Geometry check sheet. Reference: the model listing, model coordinates, mm. Face numbers are marked on the shaded views. A direction names the side the tool comes from. Coordinates: 2 decimals unless noted, no trailing zeros. Loops run counter-clockwise (first coordinate to the right, second up) from the corner with the lowest first, then second, coordinate; pieces in that order, holes last.
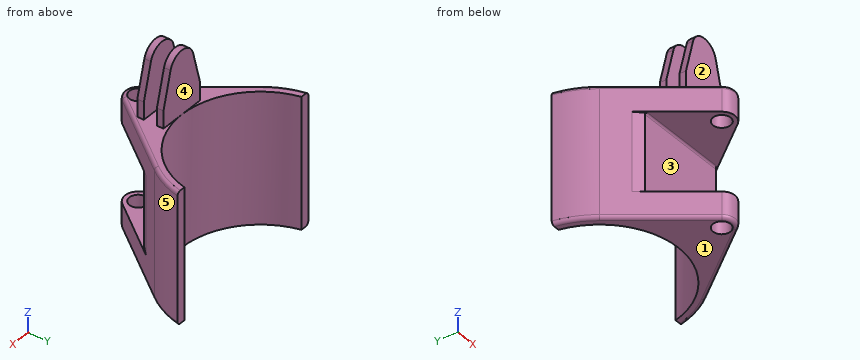
from build123d import *

# Parameters (mm, degrees)
SKETCH1_R             = 30
BOSS_EXTRUDE2_DEPTH   = 225
BOSS_EXTRUDE3_START   = 60
BOSS_EXTRUDE3_DEPTH   = 90
SKETCH3_W             = 257.405164054
SKETCH3_H             = 45
CUT_EXTRUDE1_DEPTH    = 151.9
SKETCH4_W             = 270
SKETCH4_H             = 367.4
CUT_EXTRUDE2_DEPTH    = 421.85
CHAMFER1_SIZE         = 6
CHAMFER1_SIZE2        = 32.008563289
CHAMFER1_EDGE_2_SIZE  = 6
CHAMFER1_EDGE_2_SIZE2 = 32.008563289
FILLET1_R             = 6
FILLET2_R             = 12


with BuildPart() as part:
    # Sketch1 → Boss-Extrude2 (new, symmetric)
    with BuildSketch(Plane.XY):
        with BuildLine():
            Line((238.377808514, 237.857142857), (35.756671277, -27.321428571))
            ThreePointArc((35.756671277, -27.321428571), (0, -45), (-35.756671277, -27.321428571))
            Line((-35.756671277, -27.321428571), (-238.377808514, 237.857142857))
            ThreePointArc((-238.377808514, 237.857142857), (-273.074997203, 295.782264138), (-293.938769134, 360))
            Line((-293.938769134, 360), (-263.248931622, 360))
            ThreePointArc((-263.248931622, 360), (0, 150), (263.248931622, 360))
            Line((263.248931622, 360), (293.938769134, 360))
            ThreePointArc((293.938769134, 360), (273.074997203, 295.782264138), (238.377808514, 237.857142857))
        make_face()
        Circle(SKETCH1_R, mode=Mode.SUBTRACT)
    extrude(amount=BOSS_EXTRUDE2_DEPTH, both=True)

    # Sketch2 → Boss-Extrude3 (add)
    with BuildSketch(Plane(origin=(0, 0, 0), x_dir=(1, 0, 0), z_dir=(0, 1, 0)).offset(BOSS_EXTRUDE3_START)):
        with BuildLine():
            Line((82.5, -225), (-82.5, -225))
            Line((-82.5, -225), (-82.5, -285))
            Line((-82.5, -285), (-50.709680046, -403.593320036))
            ThreePointArc((-50.709680046, -403.593320036), (0, -442.5), (50.709680046, -403.593320036))
            Line((50.709680046, -403.593320036), (82.5, -285))
            Line((82.5, -285), (82.5, -225))
        make_face()
    extrude(amount=BOSS_EXTRUDE3_DEPTH)

    # Sketch3 → Cut-Extrude1 (cut, symmetric)
    with BuildSketch(Plane(origin=(0, 0, 0), x_dir=(0, 0, -1), z_dir=(1, 0, 0))):
        with Locations((-353.702582027, 105)):
            Rectangle(SKETCH3_W, SKETCH3_H)
    extrude(amount=CUT_EXTRUDE1_DEPTH, both=True, mode=Mode.SUBTRACT)

    # Sketch4 → Cut-Extrude2 (cut, symmetric)
    with BuildSketch(Plane(origin=(0, 0, 0), x_dir=(0, 0, -1), z_dir=(1, 0, 0))):
        with Locations((0, -41.2)):
            Rectangle(SKETCH4_W, SKETCH4_H)
    extrude(amount=CUT_EXTRUDE2_DEPTH, both=True, mode=Mode.SUBTRACT)

    # Chamfer1
    chamfer1_edges = [part.edges().sort_by_distance(p)[0] for p in [
        (165.516066235, 142.5, 0),
    ]]
    chamfer1_side = [part.faces().sort_by_distance(p)[0] for p in [
        (0, 142.5, 0),
    ]]
    chamfer(chamfer1_edges, length=CHAMFER1_SIZE, length2=CHAMFER1_SIZE2, reference=chamfer1_side[0])

    # Chamfer1 edge 2
    chamfer1_edge_2_edges = [part.edges().sort_by_distance(p)[0] for p in [
        (-165.516066235, 142.5, 0),
    ]]
    chamfer1_edge_2_side = [part.faces().sort_by_distance(p)[0] for p in [
        (0, 142.5, 0),
    ]]
    chamfer(chamfer1_edge_2_edges, length=CHAMFER1_EDGE_2_SIZE, length2=CHAMFER1_EDGE_2_SIZE2, reference=chamfer1_edge_2_side[0])

    # Fillet1
    fillet1_edges = [part.edges().sort_by_distance(p)[0] for p in [
        (0, 142.5, -135),
        (0, 142.5, 135),
    ]]
    fillet(fillet1_edges, radius=FILLET1_R)

    # Fillet2
    fillet2_edges = [part.edges().sort_by_distance(p)[0] for p in [
        (273.074997203, 295.782264138, -225),
        (-273.074997203, 295.782264138, 225),
        (-137.067239895, 105.267857143, 225),
        (0, -45, 225),
        (137.067239895, 105.267857143, 225),
        (273.074997203, 295.782264138, 225),
        (137.067239895, 105.267857143, -225),
        (0, -45, -225),
        (-137.067239895, 105.267857143, -225),
        (-273.074997203, 295.782264138, -225),
    ]]
    fillet(fillet2_edges, radius=FILLET2_R)


solid = part.part
1) Access from +Z, -Z, +X, -X, +Y, -Y to the whole of each face (thin tool, end or side, straight path). Record for the marked faces 4 and 5.
Data:
face 4: +Z, +X, -X, +Y
face 5: +Z, -Z, +X, -Y
2) Section check C-C on y = 0. Count the separate pieces of the cut face and the enclosed holes in it, and give its area (3 significant figures).
Data:
separate pieces: 4
enclosed holes: 0
area: 9,430 mm2
3) Section check B-B on z = 121. Record the cut outline in (x, y), and give its area (3 significant figures).
Data:
outline: (-293.94, 360) arc R300 ccw to (-238.38, 237.86) - (-184.95, 167.93) - (-159.52, 142.5) - (159.52, 142.5) - (184.95, 167.93) - (238.38, 237.86) arc R300 ccw to (293.94, 360) - (263.25, 360) arc R270 cw to (-263.25, 360) - close
area: 22,400 mm2
4) Section check D-D on z = 315. Record the cut outline in (x, y).
Data:
outline: (-74.46, 60) - (74.46, 60) - (74.46, 82.5) - (-74.46, 82.5) - close; (-74.46, 127.5) - (74.46, 127.5) - (74.46, 150) - (-74.46, 150) - close
5) Depth check by flat-ended pin: pin 1 (6 mm diameter, centred on x = -123.5, z = 206.5, fed in from +Y); pin 2 (6 mm diameter, centred on x = -180.5, z = -124.5, fed in from +Y); pin 3 (7 mm diameter, centred on y = 142, z = 253.5, fed in from +X). Enter the tip coordinate at first touch or a pass-through.
Data:
pin 1: stops at y = 181.47
pin 2: stops at y = 221.94
pin 3: stops at x = 82.5
6) Mould release check, pull along Z, two halves, no side actions. Record for the marked faces 1, 2 and 3: +Z half, -Z half, draft (parallel to the pull), parting line (faces both ways), or undercut.
Data:
face 1: -Z half
face 2: draft
face 3: undercut
7) Material ranges on probe 1 along Y at (x, z) = (0, -163); probe 2 along Y at (x, z) = (-21, 277); probe 3 along X at (y, z) = (0, -157), recorded low to high.
Data:
probe 1: y = -45 to -30, 30 to 150
probe 2: y = 60 to 82.5, 127.5 to 150
probe 3: x = -56.63 to -30, 30 to 56.63
8) Section check A-A on z = 237.5. Record the cut outline in (x, y).
Data:
outline: (-82.5, 60) - (82.5, 60) - (82.5, 82.5) - (-82.5, 82.5) - close; (-82.5, 127.5) - (82.5, 127.5) - (82.5, 150) - (-82.5, 150) - close
